Build history of the part. All positions in model axes, mm. A direction names the side the tool comes from. Give positions to 0.01 mm unless a question says otherwise; leave off trailing zeros. Order: outer loops, then holes, each group sorted by start corner. A loop starts at its lowest first (then second) coordinate and runs counter-clockwise, first axis right, second up. Notation, with made-up numbers: M 46,-40 L 64,-40 A23 cw 64,-17 Z; hole C 16.5,22.25 d2. An arc over 180 degrees is marked long. One line per item, written item: value.
Autodesk Inventor part; units mm, degrees
ref_plane "YZ Plane" through (0, 0, 0) normal (1, 0, 0) x (0, 1, 0)
ref_plane "XZ Plane" through (0, 0, 0) normal (0, 1, 0) x (-1, 0, 0)
ref_plane "XY Plane" through (0, 0, 0) normal (0, 0, 1) x (1, 0, 0)
sketch "スケッチ1" plane through (0, 0, 0) normal (0, 1, 0) x (-1, 0, 0)
  line L0 (-12.5, 20) -> (12.5, 20)
  line L1 (12.5, 20) -> (12.5, -20)
  line L2 (12.5, -20) -> (-12.5, -20)
  line L3 (-12.5, -20) -> (-12.5, 20)
  point P0 (0, 0)
  dimension "d0" = 25
  dimension "d2" = 40
  dimension "d3" = 20
  dimension "d4" = 12.5
extrude "押し出し1" add sketch "スケッチ1" along normal blind 4
sketch "スケッチ2" plane through (0, 4, 0) normal (0, 1, 0) x (1, 0, 0)
  line L0 (-12.5, -20) -> (12.5, -20)
  line L1 (12.5, -20) -> (12.5, 20)
  line L2 (12.5, 20) -> (-12.5, 20)
  line L3 (-12.5, 20) -> (-12.5, -20)
  line L4 (-12.5, -10) -> (-10, -14.3301)
  line L5 (-10, -14.3301) -> (-10, -20)
  line L6 (10, -14.3301) -> (10, -20)
  line L7 (10, -14.3301) -> (12.5, -10)
  point P0 (0, 0)
  dimension "d7" = 20
  dimension "d9" = 2.5
  dimension "d10" = 30
  dimension "d11" = 150
  dimension "d12" = 30
  dimension "d13" = 150
extrude "押し出し2" cut sketch "スケッチ2" against normal blind 4 contours L5 L4 L3 L2 L1 L7 L6 L0 keep common part
sketch "スケッチ3" plane through (0, 4, 0) normal (0, 1, 0) x (1, 0, 0)
  line L0 (12.5, 20) -> (-12.5, 20)
  circle A0 centre (-8, 15) radius 2
  circle A1 centre (8, 15) radius 2
  point P0 (0, 0)
  dimension "d16" = 4
  dimension "d18" = 16
  dimension "d19" = 5
  dimension "d20" = 5
  dimension "d21" = 8
hole "穴1" at (-8, 4, -15) at (8, 4, -15) direction (0, -1, 0) diameter 4 end through all
sketch "スケッチ4" plane through (0, 4, 0) normal (0, 1, 0) x (1, 0, 0)
  circle A0 centre (-8, 15) radius 2
  circle A1 centre (8, 15) radius 2
  circle A2 centre (-8, 9) radius 1.5
  circle A3 centre (8, 9) radius 1.5
  circle A4 centre (-8, -6) radius 1.5
  circle A5 centre (8, -6) radius 1.5
  line L0 (12.5, 20) -> (-12.5, 20)
  point P0 (0, 0)
  dimension "d29" = 8
  dimension "d31" = 3
  dimension "d33" = 6
  dimension "d34" = 6
  dimension "d35" = 16
  dimension "d36" = 16
  dimension "d37" = 8
  dimension "d40" = 15
  dimension "d41" = 15
  dimension "d49" = 5
hole "穴2" at (-8, 4, 6) at (-8, 4, -9) at (8, 4, 6) at (8, 4, -9) direction (0, -1, 0) diameter 2.5 end through all
properties part number "Arm_Link_Shim_i"
1) Pin check, flat tips, straight feed: pin 1 (1.2 mm diameter, centred on y = 1.5, z = 17, fed in from -X); pin 2 (1.2 mm diameter, centred on y = 2, z = 16, fed in from +X). Stop position of each tip, or through.
Check values:
pin 1: x = -10
pin 2: x = 10
2) Mould opens along X. For faces 1 (the face through (11.23, 2.03, 12.2)), 2 (the face through (6, 2, -15)), 3 (the face through (-10, 2, 17)) say: released by +X, released by -X, zero draft, split by the parting line, or undercut.
Check values:
face 1: released by +X
face 2: undercut
face 3: released by -X
3) Saw through at B-B, the plane y = 1.95. Write the cut outline in (x, z).
Check values:
outline: M -12.5,-20 L 12.5,-20 L 12.5,10 L 10,14.33 L 10,20 L -10,20 L -10,14.33 L -12.5,10 Z; hole C -8,-15 d4; hole C -8,-9 d2.5; hole C -8,6 d2.5; hole C 8,-15 d4; hole C 8,-9 d2.5; hole C 8,6 d2.5
4) Drill centre lines: probe 1 along Z at (x, y) = (8, 1.1); probe 2 along X at (y, z) = (3.35, -15); probe 3 along X at (y, z) = (2.3, 6). Where is each one in solid material? Low to high. Write a range as from..to.
Check values:
probe 1: -20..-17, -13..-10.25, -7.75..4.75, 7.25..20
probe 2: -12.5..-10, -6..6, 10..12.5
probe 3: -12.5..-9.25, -6.75..6.75, 9.25..12.5
5) Saw through at D-D, the plane z = 17. Write the cut outline in (x, y).
Check values:
outline: M -10,0 L 10,0 L 10,4 L -10,4 Z
6) Saw through at A-A, the plane x = 8. Write the cut outline in (y, z).
Check values:
outline: M 0,-20 L 4,-20 L 4,-17 L 0,-17 Z; M 0,-13 L 4,-13 L 4,-10.25 L 0,-10.25 Z; M 0,-7.75 L 4,-7.75 L 4,4.75 L 0,4.75 Z; M 0,7.25 L 4,7.25 L 4,20 L 0,20 Z
7) Saw through at C-C, the plane z = -15. Write the cut outline in (x, y), then the cut area to 3 significant figures.
Check values:
outline: M -12.5,0 L -10,0 L -10,4 L -12.5,4 Z; M -6,0 L 6,0 L 6,4 L -6,4 Z; M 10,0 L 12.5,0 L 12.5,4 L 10,4 Z
area: 68.0 mm^2
8) Tool access for faces 4 (the face through (10, 2, 17)), 5 (the face through (0, 2, 20)): list every direction of +Z, -Z, +X, -X, +Y, -Y with a clear straight run to the whole face (end or side of a thin tool).
Check values:
face 4: +Z, +X, +Y, -Y
face 5: +Z, +X, -X, +Y, -Y
